```python
from build123d import *

# Parameters (mm, degrees)
SKETCH1_W           = 50
SKETCH1_H           = 21
BOSS_EXTRUDE1_DEPTH = 58
SKETCH3_R           = 7.5
CUT_EXTRUDE1_DEPTH  = 24
CUT_EXTRUDE2_REACH  = 66.025
SKETCH4_R           = 5.2
CUT_EXTRUDE3_START  = -24
SKETCH5_R           = 7.5
CUT_EXTRUDE3_DEPTH  = 24
CUT_EXTRUDE4_REACH  = 66.025
SKETCH6_R           = 4.5
CUT_EXTRUDE5_REACH  = 68.558
SKETCH8_W           = 10
SKETCH8_H           = 18
SKETCH7_R           = 4.1
CUT_EXTRUDE6_DEPTH  = 15
SKETCH11_W          = 4
SKETCH11_H          = 18
BOSS_EXTRUDE2_DEPTH = 26
SKETCH12_W          = 18
SKETCH12_H          = 18
BOSS_EXTRUDE3_DEPTH = 4
CUT_EXTRUDE7_DEPTH  = 79.487260113
FILLET1_R           = 5
FILLET2_R           = 5
FILLET3_R           = 3
SKETCH14_R          = 1.95
CUT_EXTRUDE8_DEPTH  = 10
SKETCH15_W          = 5.527864045
SKETCH15_H          = 1
CUT_EXTRUDE9_DEPTH  = 76.028327984


with BuildPart() as part:
    # Sketch1 → Boss-Extrude1 (new body)
    with BuildSketch(Plane(origin=(0, 0, 0), x_dir=(1, 0, 0), z_dir=(0, 1, 0))):
        Rectangle(SKETCH1_W, SKETCH1_H)
    extrude(amount=BOSS_EXTRUDE1_DEPTH)

    # Sketch3 → Cut-Extrude1 (cut)
    with BuildSketch(Plane(origin=(0, 58, 0), x_dir=(1, 0, 0), z_dir=(0, 1, 0))):
        with Locations(Location((-15, 0, 0), (0, 0, 270))):
            Circle(SKETCH3_R)
    extrude(amount=-CUT_EXTRUDE1_DEPTH, mode=Mode.SUBTRACT)

    # Sketch4 → Cut-Extrude2 (cut, up to next)
    with BuildSketch(Plane(origin=(0, 58, 0), x_dir=(1, 0, 0), z_dir=(0, 1, 0)), mode=Mode.PRIVATE) as cut_extrude2_sk1:
        with Locations(Location((15, 0, 0), (0, 0, 270))):
            Circle(SKETCH4_R)
    cut_extrude2_tool1 = extrude(cut_extrude2_sk1.sketch, amount=-CUT_EXTRUDE2_REACH, mode=Mode.PRIVATE) & part.part
    add(cut_extrude2_tool1.solids().sort_by_distance((15, 58, 0))[0], mode=Mode.SUBTRACT)

    # Sketch5 → Cut-Extrude3 (cut)
    with BuildSketch(Plane.XZ.offset(CUT_EXTRUDE3_START)):
        with Locations(Location((-15, 0, 0), (0, 0, 90))):
            Circle(SKETCH5_R)
    extrude(amount=CUT_EXTRUDE3_DEPTH, mode=Mode.SUBTRACT)

    # Sketch6 → Cut-Extrude4 (cut, up to next)
    with BuildSketch(Plane.XZ, mode=Mode.PRIVATE) as cut_extrude4_sk1:
        with Locations(Location((-15, 0, 0), (0, 0, 270))):
            Circle(SKETCH6_R)
    cut_extrude4_tool1 = extrude(cut_extrude4_sk1.sketch, amount=-CUT_EXTRUDE4_REACH, mode=Mode.PRIVATE) & part.part
    add(cut_extrude4_tool1.solids().sort_by_distance((-15, 0, 0))[0], mode=Mode.SUBTRACT)

    # Sketch8 → Cut-Extrude5 (cut, up to next)
    with BuildSketch(Plane.XY.offset(10.5), mode=Mode.PRIVATE) as cut_extrude5_sk1:
        with Locations((0, 29)):
            Rectangle(SKETCH8_W, SKETCH8_H)
    cut_extrude5_tool1 = extrude(cut_extrude5_sk1.sketch, amount=-CUT_EXTRUDE5_REACH, mode=Mode.PRIVATE) & part.part
    add(cut_extrude5_tool1.solids().sort_by_distance((0, 29, 10.5))[0], mode=Mode.SUBTRACT)

    # Sketch7 → Cut-Extrude6 (cut)
    with BuildSketch(Plane.XY.offset(10.5)):
        with Locations((0, 49)):
            Circle(SKETCH7_R)
        with Locations(Location((0, 9, 0), (0, 0, 180))):
            Circle(SKETCH7_R)
    extrude(amount=-CUT_EXTRUDE6_DEPTH, mode=Mode.SUBTRACT)

    # Sketch11 → Boss-Extrude2 (add)
    with BuildSketch(Plane(origin=(0, 0, -10.5), x_dir=(-1, 0, 0), z_dir=(0, 0, -1))):
        with Locations((7, 29)):
            Rectangle(SKETCH11_W, SKETCH11_H)
        with Locations((-7, 29)):
            Rectangle(SKETCH11_W, SKETCH11_H)
    extrude(amount=BOSS_EXTRUDE2_DEPTH)

    # Sketch12 → Boss-Extrude3 (add)
    with BuildSketch(Plane(origin=(0, 0, -36.5), x_dir=(-1, 0, 0), z_dir=(0, 0, -1))):
        with Locations((0, 29)):
            Rectangle(SKETCH12_W, SKETCH12_H)
    extrude(amount=BOSS_EXTRUDE3_DEPTH)

    # Sketch13 → Cut-Extrude7 (cut, through all)
    with BuildSketch(Plane(origin=(9, 0, 0), x_dir=(0, 0, -1), z_dir=(1, 0, 0))):
        with BuildLine():
            Line((16.25, 31.75), (25.25, 31.75))
            ThreePointArc((25.25, 31.75), (28, 29), (25.25, 26.25))
            Line((25.25, 26.25), (16.25, 26.25))
            ThreePointArc((16.25, 26.25), (13.5, 29), (16.25, 31.75))
        make_face()
    extrude(amount=-CUT_EXTRUDE7_DEPTH, mode=Mode.SUBTRACT)

    # Fillet1
    fillet1_edges = [part.edges().sort_by_distance(p)[0] for p in [
        (25, 29, 10.5),
        (-25, 29, 10.5),
    ]]
    fillet(fillet1_edges, radius=FILLET1_R)

    # Fillet2
    fillet2_edges = [part.edges().sort_by_distance(p)[0] for p in [
        (-7, 38, -10.5),
        (-7, 20, -10.5),
        (7, 20, -10.5),
        (7, 38, -10.5),
    ]]
    fillet(fillet2_edges, radius=FILLET2_R)

    # Fillet3
    fillet3_edges = [part.edges().sort_by_distance(p)[0] for p in [
        (-5, 29, -36.5),
        (5, 29, -36.5),
        (-9, 29, -40.5),
        (9, 29, -40.5),
    ]]
    fillet(fillet3_edges, radius=FILLET3_R)

    # Sketch14 → Cut-Extrude8 (cut)
    with BuildSketch(Plane.XZ):
        with Locations(Location((20.550788232, 5.550788232, 0), (0, 0, 270))):
            Circle(SKETCH14_R)
        with Locations(Location((9.449211768, -5.550788232, 0), (0, 0, 270))):
            Circle(SKETCH14_R)
    extrude(amount=-CUT_EXTRUDE8_DEPTH, mode=Mode.SUBTRACT)

    # Sketch15 → Cut-Extrude9 (cut, through all)
    with BuildSketch(Plane(origin=(0, 58, 0), x_dir=(1, 0, 0), z_dir=(0, 1, 0))):
        with Locations((-22.236067977, 0)):
            Rectangle(SKETCH15_W, SKETCH15_H)
    extrude(amount=-CUT_EXTRUDE9_DEPTH, mode=Mode.SUBTRACT)


solid = part.part
```
The model under review builds one solid part; all positions refer to its coordinate system, in mm. A direction names the side the tool comes from. Round coordinates to 2 decimals unless told otherwise and drop trailing zeros. Order: outer loops, then holes, each group sorted by start corner. A loop starts at its lowest first (then second) coordinate and runs counter-clockwise, first axis right, second up. Notation, with made-up numbers: (1.25, 47) - (22.25, 47) arc R27 cw to (22.25, 63) - close; hole circle Ø11 at (89, -27). An arc over 180 degrees is marked (long way). Answer in a Markdown table with one row per item.
(1) Take a section at B-B on z = -21.5. Write out the cut boundary in (x, y), plus the area to 3 significant figures.
Result set:
| item | result |
|---|---|
| outline | (-9, 20) - (-5, 20) - (-5, 26.25) - (-9, 26.25) - close; (-9, 31.75) - (-5, 31.75) - (-5, 38) - (-9, 38) - close; (5, 20) - (9, 20) - (9, 26.25) - (5, 26.25) - close; (5, 31.75) - (9, 31.75) - (9, 38) - (5, 38) - close |
| area | 100 mm2 |
(2) Clearance check with flat-ended pins moving along their axes: P1, Ø4.5, axis at x = -23, y = 38.5, coming from the +Z side; P2, Ø3, axis at x = -0.5, y = 32.5, coming from the +Z side; P3, Ø9, axis at x = 1, z = -28.5, coming from the +Y side. State where each tip first meets the part, or that it passes through.
Result set:
| item | result |
|---|---|
| P1 | stops at z = 10.44 |
| P2 | stops at z = -36.5 |
| P3 | stops at y = 38 |
(3) Machinability: for faces 1 (the face through (4.1, 29.13, -35.64)), 2 (the face through (-3.022, 51.771, 3.105)), 3 (the face through (9, 10, -6)), 4 (the face through (-7, 28.9, -13.5)), which of the approach directions +Z, -Z, +X, -X, +Y, -Y give a long, thin tool a straight path to every point of the face, cutting with its end or side? Answer none if there is none.
Result set:
| item | result |
|---|---|
| face 1 | +Z, +Y, -Y |
| face 2 | +Z |
| face 3 | -Y |
| face 4 | +X, -X |
(4) Mouldability with a two-part tool opening along Y and no side actions: class faces 5 (the face through (7, 28.9, -13.5)), 6 (the face through (23.57, 29.41, 9)), 7 (the face through (-7, 26.25, -21)), 8 (the face through (-10, 24, 0)) as released by +Y, released by -Y, zero draft, split by the parting line, or undercut.
Result set:
| item | result |
|---|---|
| face 5 | undercut |
| face 6 | zero draft |
| face 7 | undercut |
| face 8 | released by -Y |
(5) For line 1 (X direction, y = 27.5, z = 0); line 2 (X direction, y = 33.5, z = -21); line 3 (X direction, y = 42.5, z = 0), list the stretches that pass through material, from the lowest coordinate up. Write a range as from..to.
Result set:
| item | result |
|---|---|
| line 1 | x = -10.5..-5, 5..9.8, 20.2..25 |
| line 2 | x = -9..-5, 5..9 |
| line 3 | x = -7.5..9.8, 20.2..25 |
(6) Take a section at A-A on y = 29. Count the separate pieces of the cut face and the enclosed holes in it, plus the area to 3 significant figures.
Result set:
| item | result |
|---|---|
| separate pieces | 3 |
| enclosed holes | 1 |
| area | 839 mm2 |
(7) Take a section at C-C on x = 15. Write out the cut boundary in (y, z), plus the area to 3 significant figures.
Result set:
| item | result |
|---|---|
| outline | (0, -10.5) - (58, -10.5) - (58, -5.2) - (0, -5.2) - close; (0, 5.2) - (58, 5.2) - (58, 10.5) - (0, 10.5) - close |
| area | 615 mm2 |
(8) Take a section at D-D on z = -12. Write out the cut boundary in (x, y).
Result set:
| item | result |
|---|---|
| outline | (-9, 18.57) - (-5, 18.57) - (-5, 39.43) - (-9, 39.43) - close; (5, 18.57) - (9, 18.57) - (9, 39.43) - (5, 39.43) - close |
